Verification items for the finished model (mm, model axes). Face numbers are marked on the shaded views. A direction names the side the tool comes from. Round coordinates to 2 decimals unless told otherwise and drop trailing zeros. Order: outer loops, then holes, each group sorted by start corner. A loop starts at its lowest first (then second) coordinate and runs counter-clockwise, first axis right, second up. Notation, with made-up numbers: (70.25, -30) -> (80.25, -30) arc R11 cw to (80.25, -15) -> close; hole circle Ø7 at (-31, -21). An arc over 180 degrees is marked (long way). Put each result on its own line as item: value.
from build123d import *

# Parameters (mm, degrees)
SKETCH1_R           = 2.5
BOSS_EXTRUDE1_DEPTH = 12
SKETCH2_R           = 2.5
BOSS_EXTRUDE2_DEPTH = 25


with BuildPart() as part:
    # Sketch1 → Boss-Extrude1 (new body)
    with BuildSketch(Plane(origin=(0, 0, 0), x_dir=(1, 0, 0), z_dir=(0, 1, 0))):
        with Locations(Location((0, 0, 0), (0, 0, 270))):
            Circle(SKETCH1_R)
    extrude(amount=BOSS_EXTRUDE1_DEPTH)

    # Sketch2 → Boss-Extrude2 (add, symmetric)
    with BuildSketch(Plane.XY):
        with Locations((0, 6)):
            Circle(SKETCH2_R)
    extrude(amount=BOSS_EXTRUDE2_DEPTH, both=True)


solid = part.part
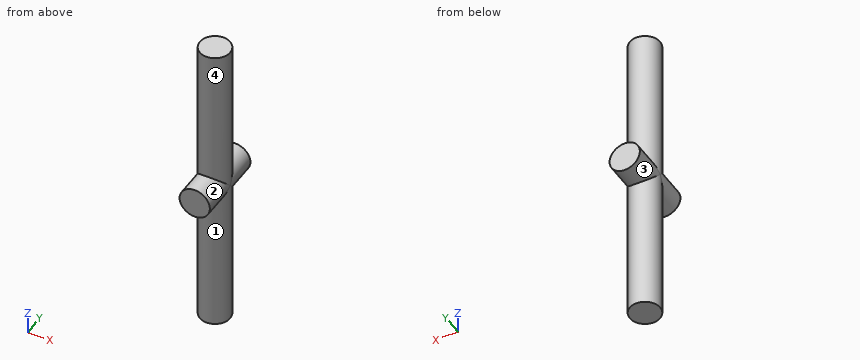
Item 1: Section check B-B on y = 5. Record the boundary of the cut face in (x, z).
Check sheet entries:
outline: (-2.29, -25) -> (2.29, -25) -> (2.29, -1) arc R2.5 ccw to (2.29, 1) -> (2.29, 25) -> (-2.29, 25) -> (-2.29, 1) arc R2.5 ccw to (-2.29, -1) -> close
Item 2: Section check C-C on x = 0. Record the boundary of the cut face in (y, z), then the cut area to 3 significant figures.
Check sheet entries:
outline: (0, -2.5) -> (3.5, -2.5) -> (3.5, -25) -> (8.5, -25) -> (8.5, -2.5) -> (12, -2.5) -> (12, 2.5) -> (8.5, 2.5) -> (8.5, 25) -> (3.5, 25) -> (3.5, 2.5) -> (0, 2.5) -> close
area: 285 mm^2
Item 3: Material ranges on L1, parallel to Z at x = 0.1, y = 10.75; L2, parallel to X at y = 6.5, z = -20.5; L3, parallel to Z at x = -1.7, y = 9.25, recorded low to high. Write a range as [from, to].
Check sheet entries:
L1: z = [-2.5, 2.5]
L2: x = [-2.45, 2.45]
L3: z = [-1.83, 1.83]
Item 4: Tool access check on the marked faces 1, 2, 3 and 4. Record the directions out of +Z, -Z, +X, -X, +Y, -Y that give a thin tool (end or side, any length) a straight path to the whole face; none if there is none.
Check sheet entries:
face 1: -Z
face 2: -Y
face 3: +Y
face 4: +Z
Item 5: Gauge pin test, flat ends, axial feed: pin 1 Ø2 at (x, y) = (-1, 3) entering from -Z; pin 2 Ø3 at (x, y) = (-1, 10) entering from +Z; pin 3 Ø2 at (x, z) = (1.5, -9) entering from +Y; pin 4 Ø2 at (x, z) = (1, -4.5) entering from +Y. Record the tip position at first contact, or that the pin passes through.
Check sheet entries:
pin 1: stops at z = -25
pin 2: stops at z = 2.5
pin 3: stops at y = 8.45
pin 4: stops at y = 8.5
Item 6: Section check D-D on z = 13. Record the boundary of the cut face in (x, y).
Check sheet entries:
outline: circle Ø5 at (0, 6)
Item 7: Section check A-A on x = 2. Record the boundary of the cut face in (y, z).
Check sheet entries:
outline: (0, -1.5) -> (4.5, -1.5) -> (4.5, -25) -> (7.5, -25) -> (7.5, -1.5) -> (12, -1.5) -> (12, 1.5) -> (7.5, 1.5) -> (7.5, 25) -> (4.5, 25) -> (4.5, 1.5) -> (0, 1.5) -> close
